Can you work these out from the model? Positions are in its coordinate system, mm. A direction names the side the tool comes from. Give positions to 0.01 mm unless a question says otherwise; leave off trailing zeros. Write each loop counter-clockwise with the first axis right and the second up, starting at its lowest first coordinate (ties: lowest second). Pieces come first, ordered by that corner, then holes.
from build123d import *

# Parameters (mm, degrees)
F0_W      = 1778
F0_H      = 1016
F0_R      = 254
F1_DEPTH  = 508
F2_R      = 254
F3_W      = 254
F3_H      = 1016
F4_DEPTH  = 508
F5_W      = 508
F5_H      = 254
F6_DEPTH  = 508
F7_W      = 508
F7_H      = 254
F8_DEPTH  = 508
F10_DEPTH = 254


with BuildPart() as f1:
    # F0 (on Top) → F1 (new body)
    with BuildSketch(Plane.XY):
        with Locations((-829.280311, 467.563289)):
            Rectangle(F0_W, F0_H)
        with Locations((-412.175477, 538.300574)):
            Circle(F0_R, mode=Mode.SUBTRACT)
    extrude(amount=F1_DEPTH)

    # F2
    f2_edges = [f1.edges().sort_by_distance(p)[0] for p in [
        (59.719689, -40.436711, 254),
        (59.719689, 975.563289, 254),
    ]]
    fillet(f2_edges, radius=F2_R)

    # F3 (on face) → F4 (join)
    with BuildSketch(Plane.XY.offset(508)):
        with Locations((-1591.280311, 467.563289)):
            Rectangle(F3_W, F3_H)
    extrude(amount=F4_DEPTH)

    # F5 (on face) → F6 (join)
    with BuildSketch(Plane.XY.offset(508)):
        with Locations((-1210.280311, 848.563289)):
            Rectangle(F5_W, F5_H)
    extrude(amount=F6_DEPTH)

    # F7 (on face) → F8 (join)
    with BuildSketch(Plane.XY.offset(508)):
        with Locations((-1210.280311, 86.563289)):
            Rectangle(F7_W, F7_H)
    extrude(amount=F8_DEPTH)

    # F9 (on face) → F10 (cut)
    with BuildSketch(Plane.XZ.offset(40.436711)):
        Polygon((-1464.280311, 1016), (-956.280311, 508), (-956.280311, 1016), align=None)
    extrude(amount=-F10_DEPTH, mode=Mode.SUBTRACT)


solid = f1.part
(1) Imagine slicing it at A-A, the plane y = 661.5. Write out the boundary of the cut face in (x, z).
Returned:
outline: (-1718.28, 0) - (-634.3, 0) - (-634.3, 508) - (-1464.28, 508) - (-1464.28, 1016) - (-1718.28, 1016) - close; (-190.05, 0) - (59.72, 0) - (59.72, 508) - (-190.05, 508) - close
(2) Imagine slicing it at D-D, the plane x = -267. Write out the boundary of the cut face in (y, z), plus the area to 3 significant figures.
Returned:
outline: (-40.44, 0) - (329.88, 0) - (329.88, 508) - (-40.44, 508) - close; (746.72, 0) - (975.56, 0) - (975.56, 508) - (746.72, 508) - close
area: 304,000 mm2
(3) For faces 4 (the face through (-956.28, 847, 758)), 5 (the face through (-1214, 721.563, 758)), 6 (the face through (-1213.84, 84.79, 765.56)), 7 (the face through (-445.24, 790.14, 250.44)), which set-ups out of +Z, -Z, +X, -X, +Y, -Y let a thin tool reach every point of the face, with its end or its side?
Returned:
face 4: +Z, +X, +Y, -Y
face 5: +Z, +X
face 6: +Z, +X, -Y
face 7: +Z, -Z
(4) Imagine slicing it at C-C, the plane z = 149. Write out the boundary of the cut face in (x, y).
Returned:
outline: (-1718.28, -40.44) - (-194.28, -40.44) arc R254 ccw to (59.72, 213.56) - (59.72, 721.56) arc R254 ccw to (-194.28, 975.56) - (-1718.28, 975.56) - close; hole circle Ø508 at (-412.18, 538.3)
(5) If we mould it in two halves opening along Y, with no side actions, what happens to faces 1 (the face through (-1136, -40.437, 388)), 2 (the face through (-713, 475, 508)), 3 (the face through (-842, 475, 0))? For each: +Y half, -Y half, draft (parallel to the pull), parting line (faces both ways), or undercut.
Returned:
face 1: -Y half
face 2: undercut
face 3: draft
(6) Imagine slicing it at B-B, the plane x = -1288. Write out the boundary of the cut face in (y, z), plus the area to 3 significant figures.
Returned:
outline: (-40.44, 0) - (975.56, 0) - (975.56, 1016) - (721.56, 1016) - (721.56, 508) - (213.56, 508) - (213.56, 839.72) - (-40.44, 839.72) - close
area: 729,000 mm2
(7) Will these pins go through, and if not, where does the flat tip stop? P1, Ø6, axis at x = -1053, y = 662.5, coming from the -Z side; P2, Ø2, axis at x = -788.5, y = 735.5, coming from the +Z side; P3, Ø8, axis at y = 819, z = 151, coming from the +X side.
Returned:
P1: stops at z = 0
P2: stops at z = 508
P3: stops at x = 41.91
(8) If I drill on L1, parallel to X at y = 546, z = 215.5; L2, parallel to Z at x = -814, y = 345.5; L3, parallel to Y at x = -1043, z = 936, over which ranges is the centre line in solid material (lowest first)?
Returned:
L1: x = -1718.28 to -666.06, -158.29 to 59.72
L2: z = 0 to 508
L3: y = 721.56 to 975.56
